Design review of the part built by this model. Coordinates are the model's own, in mm. A direction names the side the tool comes from. Give positions to 0.01 mm unless a question says otherwise; leave off trailing zeros. Loops run counter-clockwise (first coordinate to the right, second up) from the corner with the lowest first, then second, coordinate; pieces in that order, holes last. Notation, with made-up numbers: (-29, 79) -> (23, 79) arc R23 cw to (23, 112) -> close; hole circle Ø2 at (59.25, -21). An arc over 180 degrees is marked (long way). Answer in a Markdown table with one row per item. Add a question column.
(1) For line 1 (Y direction, x = -118, z = 17); line 2 (X direction, y = 27, z = 52); line 3 (Z direction, x = -44, y = 18), list the stretches that pass through material, from the lowest coordinate up.
(2) Consider section B-B on y = 48. Write out the cut boundary in (x, z), then the cut area to 3 significant figures.
(3) Consider section A-A on z = 28. Write out the cut boundary in (x, y).
(4) Draft analysis for pull direction Y (two halves, no side actions). For faces 3 (the flat face through (-84, 0, 27)), 4 (the flat face through (-86, 45, 5)), 5 (the flat face through (-170, 44, 27)), state which applies: +Y half, -Y half, draft (parallel to the pull), parting line (faces both ways), or undercut.
(5) Consider section C-C on x = -139. Write out the cut boundary in (y, z).
(6) For faces 1 (the flat face through (-84, 90, 27)), 2 (the flat face through (-165, 45, 33)), list the 3-axis set-ups (+Z, -Z, +X, -X, +Y, -Y) from which the entire face can be reached by the end or side of a thin tool; tool diameter is ignored.
(7) For pin 1 (19 mm diameter, centred on x = -104.5, y = 33.5, fed in from +Z); pin 2 (5 mm diameter, centred on x = -71, y = 12, fed in from +Z), all flat-tipped, find the tip position at first contact; note any pin that passes through.
from build123d import *

# Parameters (mm, degrees)
IZIM1_W                     = 80
IZIM1_H                     = 160
Y_KSEKLIK_EKSTR_ZYON1_DEPTH = 5
IZIM1_3_W                   = 90
IZIM1_3_H                   = 170
IZIM1_3_W_2                 = 80
IZIM1_3_H_2                 = 160
Y_KSEKLIK_EKSTR_ZYON2_DEPTH = 55
RADYUS2_R                   = 8
RADYUS4_R                   = 2


with BuildPart() as part:
    # Çizim1 → Yükseklik-Ekstrüzyon1 (new body)
    with BuildSketch(Plane(origin=(0, 0, 0), x_dir=(0, 1, 0), z_dir=(0, 0, 1))):
        with Locations((45, 85)):
            Rectangle(IZIM1_W, IZIM1_H)
    extrude(amount=Y_KSEKLIK_EKSTR_ZYON1_DEPTH)

    # Çizim1<3> → Yükseklik-Ekstrüzyon2 (add)
    with BuildSketch(Plane(origin=(0, 0, 0), x_dir=(0, 1, 0), z_dir=(0, 0, 1))):
        with Locations((45, 85)):
            Rectangle(IZIM1_3_W, IZIM1_3_H)
        with Locations((45, 85)):
            Rectangle(IZIM1_3_W_2, IZIM1_3_H_2, mode=Mode.SUBTRACT)
    extrude(amount=Y_KSEKLIK_EKSTR_ZYON2_DEPTH)

    # Radyus2
    radyus2_edges = [part.edges().sort_by_distance(p)[0] for p in [
        (-165, 45, 5),
        (-5, 85, 30),
        (-165, 85, 30),
        (-165, 5, 30),
        (-5, 5, 30),
        (-85, 5, 5),
        (-5, 45, 5),
        (-85, 85, 5),
    ]]
    fillet(radyus2_edges, radius=RADYUS2_R)

    # Radyus4
    radyus4_edges = [part.edges().sort_by_distance(p)[0] for p in [
        (-85, 5, 55),
        (-5, 45, 55),
        (-85, 85, 55),
        (-165, 45, 55),
        (-7.343145751, 7.343145751, 55),
        (-7.343145751, 82.656854249, 55),
        (-162.656854249, 82.656854249, 55),
        (-162.656854249, 7.343145751, 55),
    ]]
    fillet(radyus4_edges, radius=RADYUS4_R)


solid = part.part
Values follow:
| question | item | result |
|---|---|---|
| 1 | line 1 | 0 to 5, 85 to 90 |
| 1 | line 2 | -170 to -165, -5 to 0 |
| 1 | line 3 | 0 to 5 |
| 2 | outline | (-170, 0) -> (0, 0) -> (0, 55) -> (-3, 55) arc R2 ccw to (-5, 53) -> (-5, 13) arc R8 cw to (-13, 5) -> (-157, 5) arc R8 cw to (-165, 13) -> (-165, 53) arc R2 ccw to (-167, 55) -> (-170, 55) -> close |
| 2 | area | 1,380 mm2 |
| 3 | outline | (-170, 0) -> (0, 0) -> (0, 90) -> (-170, 90) -> close; hole (-165, 13) arc R8 ccw to (-157, 5) -> (-13, 5) arc R8 ccw to (-5, 13) -> (-5, 77) arc R8 ccw to (-13, 85) -> (-157, 85) arc R8 ccw to (-165, 77) -> close |
| 4 | face 3 | -Y half |
| 4 | face 4 | undercut |
| 4 | face 5 | draft |
| 5 | outline | (0, 0) -> (90, 0) -> (90, 55) -> (87, 55) arc R2 ccw to (85, 53) -> (85, 13) arc R8 cw to (77, 5) -> (13, 5) arc R8 cw to (5, 13) -> (5, 53) arc R2 ccw to (3, 55) -> (0, 55) -> close |
| 6 | face 1 | +Z, -Z, +X, -X, +Y |
| 6 | face 2 | +Z |
| 7 | pin 1 | z = 5 |
| 7 | pin 2 | z = 5.81 |
